```python
from build123d import *

# Parameters (mm, degrees)
SKETCH1_R           = 3.4
SKETCH1_R_2         = 1
SKETCH1_R_3         = 1.5
BOSS_EXTRUDE1_DEPTH = 1.2
FILLET1_R           = 2


with BuildPart() as part:
    # Sketch1 → Boss-Extrude1 (new body)
    with BuildSketch(Plane.XY):
        with BuildLine():
            Line((8.886327877, -1.425895111), (5, -25.645898034))
            ThreePointArc((5, -25.645898034), (8.80624304, -31.091650066), (2.5, -29))
            ThreePointArc((2.5, -29), (0, -26.5), (-2.5, -29))
            ThreePointArc((-2.5, -29), (-8.80624304, -31.091650066), (-5, -25.645898034))
            Line((-5, -25.645898034), (-8.886327877, -1.425895111))
            ThreePointArc((-8.886327877, -1.425895111), (0, 9), (8.886327877, -1.425895111))
        make_face()
        Circle(SKETCH1_R, mode=Mode.SUBTRACT)
        with Locations((0, 6.2)):
            Circle(SKETCH1_R_2, mode=Mode.SUBTRACT)
        with Locations((6.2, 0)):
            Circle(SKETCH1_R_2, mode=Mode.SUBTRACT)
        with Locations((0, -6.2)):
            Circle(SKETCH1_R_2, mode=Mode.SUBTRACT)
        with Locations((-6.2, 0)):
            Circle(SKETCH1_R_2, mode=Mode.SUBTRACT)
        with Locations((6, -29)):
            Circle(SKETCH1_R_3, mode=Mode.SUBTRACT)
        with Locations(Location((-6, -29, 0), (0, 0, 180))):
            Circle(SKETCH1_R_3, mode=Mode.SUBTRACT)
        with BuildLine():
            Line((4.861419119, -7.574074475), (2.795583653, -20.448577761))
            ThreePointArc((2.795583653, -20.448577761), (0, -22.831344198), (-2.795583653, -20.448577761))
            Line((-2.795583653, -20.448577761), (-4.861419119, -7.574074475))
            ThreePointArc((-4.861419119, -7.574074475), (0, -9), (4.861419119, -7.574074475))
        make_face(mode=Mode.SUBTRACT)
    extrude(amount=BOSS_EXTRUDE1_DEPTH)

    # Fillet1
    fillet1_edges = [part.edges().sort_by_distance(p)[0] for p in [
        (5, -25.645898034, 0.6),
        (-5, -25.645898034, 0.6),
        (4.861419119, -7.574074475, 0.6),
        (-4.861419119, -7.574074475, 0.6),
    ]]
    fillet(fillet1_edges, radius=FILLET1_R)


solid = part.part
```
CAD build for the part. Positions are in the model's coordinates, mm. A direction names the side the tool comes from. Coordinates: 2 decimals unless noted, no trailing zeros. Order: outer loops, then holes, each group sorted by start corner. A loop starts at its lowest first (then second) coordinate and runs counter-clockwise, first axis right, second up. Notation, with made-up numbers: M 38.25,27.5 L 69.25,27.5 A5 ccw 69.25,32.5 Z; hole C 13.25,2 d1. An arc over 180 degrees is marked long. Answer as CSV lines item,"result".
1) Cut at D-D (x = 6). List the corners of the cut face in (y, z), then the cut area to 3 significant figures.
Verdict:
outline,"M -32.5,0 L -30.5,0 L -30.5,1.2 L -32.5,1.2 Z; M -27.5,0 L -25.15,0 L -25.15,1.2 L -27.5,1.2 Z; M -19.41,0 L -0.98,0 L -0.98,1.2 L -19.41,1.2 Z; M 0.98,0 L 6.71,0 L 6.71,1.2 L 0.98,1.2 Z"
area,"34.2 mm2"
2) Cut at C-C (z = 0.7). Give the number of separate pieces and of enclosed holes in the cut face, then the cut area to 3 significant figures.
Verdict:
separate pieces,"1"
enclosed holes,"8"
area,"422 mm2"
3) Drill centre lines: L1, parallel to X at y = -28, z = 1.15; L2, parallel to Y at x = -1.25, z = 1.15; L3, parallel to Y at x = -0.75, z = 1.15. Where is each one in solid material? Low to high. Write a range as from..to.
Verdict:
L1,"-9.35..-7.12, -4.88..-2.29, 2.29..4.88, 7.12..9.35"
L2,"-26.83..-22.54, -8.91..-3.16, 3.16..8.91"
L3,"-26.62..-22.73, -8.97..-6.86, -5.54..-3.32, 3.32..5.54, 6.86..8.97"
4) Cut at A-A (y = -9.5). List the corners of the cut face in (x, z).
Verdict:
outline,"M -7.59,0 L -3.89,0 L -3.89,1.2 L -7.59,1.2 Z; M 3.89,0 L 7.59,0 L 7.59,1.2 L 3.89,1.2 Z"
5) Mould opens along Y. For faces 4 (the cylindrical face through (-5.805, -30.487, 0.592)), 5 (the cylindrical face through (0.1, -26.5, 0.6)), 6 (the flat face through (2, -7, 0)) say: released by +Y, released by -Y, zero draft, split by the parting line, or undercut.
Verdict:
face 4,"undercut"
face 5,"released by -Y"
face 6,"zero draft"
6) Cut at B-B (x = 0). List the corners of the cut face in (y, z).
Verdict:
outline,"M -26.5,0 L -22.83,0 L -22.83,1.2 L -26.5,1.2 Z; M -9,0 L -7.2,0 L -7.2,1.2 L -9,1.2 Z; M -5.2,0 L -3.4,0 L -3.4,1.2 L -5.2,1.2 Z; M 3.4,0 L 5.2,0 L 5.2,1.2 L 3.4,1.2 Z; M 7.2,0 L 9,0 L 9,1.2 L 7.2,1.2 Z"
7) 3-axis set-ups, long thin cutter, end or side, ignore diameter. For faces 1 (the flat face through (7.152, -12.234, 0.592)), 2 (the flat face through (3.56, -15.69, 0.59)), 3 (the cylindrical face through (-5.66, -24.75, 0.61)): which of +Z, -Z, +X, -X, +Y, -Y reach the whole face in a straight line?
Verdict:
face 1,"+Z, -Z, +X"
face 2,"+Z, -Z"
face 3,"+Z, -Z, -X"
8) Flat gauge pin, fed straight in: P1, Ø1.2, axis at x = 0, y = 6.2, coming from the -Z side. Where does the tip first touch, or does it go through?
Verdict:
P1,"through"
